```python
from build123d import *

# Parameters (mm, degrees)
BOSS_EXTRUDE1_DEPTH  = 40
SKETCH3_R            = 9
CUT_EXTRUDE1_DEPTH   = 135.350288425
SKETCH4_W            = 25
SKETCH4_H            = 30
CUT_EXTRUDE2_DEPTH   = 30
SKETCH5_R            = 11.1
CUT_EXTRUDE3_DEPTH   = 7
SKETCH6_R            = 11.1
CUT_EXTRUDE4_DEPTH   = 7
CUT_EXTRUDE5_DEPTH   = 41
SKETCH9_W            = 50
SKETCH9_H            = 40
BOSS_EXTRUDE2_DEPTH  = 30
SKETCH11_R           = 1.45
CUT_EXTRUDE8_DEPTH   = 20
SKETCH15_W           = 81.391173049
SKETCH15_H           = 40
SKETCH15_W_2         = 77.391173049
SKETCH15_H_2         = 36
CUT_EXTRUDE9_DEPTH   = 4
SKETCH16_W           = 30
SKETCH16_H           = 40
SKETCH16_W_2         = 26
SKETCH16_H_2         = 36
CUT_EXTRUDE10_DEPTH  = 4
CUT_EXTRUDE11_DEPTH  = 41
SKETCH18_W           = 153.620263659
SKETCH18_H           = 20
BOSS_EXTRUDE3_DEPTH  = 40
CUT_EXTRUDE7_DEPTH   = 41
SKETCH19_W           = 15
SKETCH19_H           = 15
CUT_EXTRUDE12_DEPTH  = 150
SKETCH20_R           = 1.45
CUT_EXTRUDE13_DEPTH  = 20
CUT_EXTRUDE16_DEPTH  = 3
CUT_EXTRUDE18_START  = -7
CUT_EXTRUDE18_DEPTH  = 2.55
SKETCH38_W           = 90
SKETCH38_H           = 20
CUT_EXTRUDE19_DEPTH  = 45.5
CUT_EXTRUDE21_START  = -31.810131
CUT_EXTRUDE21_DEPTH  = 90
BOSS_EXTRUDE11_DEPTH = 40
CHAMFER1_SIZE        = 1.5


with BuildPart() as part:
    # Sketch1 → Boss-Extrude1 (new body)
    with BuildSketch(Plane(origin=(0, 0, 0), x_dir=(1, 0, 0), z_dir=(0, 1, 0))):
        Polygon((-79.503540842, -54.434705768), (-79.503540842, -4.434705768), (-46.700027791, 28.368807283), (-21.951290449, 53.117544624), (-14.880222638, 46.046476813), (-43.164493885, 17.762205565), (-14.880222638, -10.522065682), (13.40404861, 17.762205565), (60.496459158, -29.330204983), (60.496459158, -54.434705768), align=None)
    extrude(amount=BOSS_EXTRUDE1_DEPTH)

    # Sketch3 → Cut-Extrude1 (cut, through all)
    with BuildSketch(Plane(origin=(-37.534417537, 0, -37.534417537), x_dir=(-0.707106781, 0, 0.707106781), z_dir=(-0.707106781, 0, -0.707106781))):
        with Locations((-7.037869671, 20)):
            Circle(SKETCH3_R)
    extrude(amount=-CUT_EXTRUDE1_DEPTH, mode=Mode.SUBTRACT)

    # Sketch4 → Cut-Extrude2 (cut)
    with BuildSketch(Plane(origin=(15.583127088, 0, -15.583127088), x_dir=(-0.707106781, 0, -0.707106781), z_dir=(0.707106781, 0, -0.707106781))):
        with Locations((-19.418317664, 20)):
            Rectangle(SKETCH4_W, SKETCH4_H)
    extrude(amount=-CUT_EXTRUDE2_DEPTH, mode=Mode.SUBTRACT)

    # Sketch5 → Cut-Extrude3 (cut)
    with BuildSketch(Plane(origin=(-37.534417537, 0, -37.534417537), x_dir=(-0.707106781, 0, 0.707106781), z_dir=(-0.707106781, 0, -0.707106781))):
        with Locations((-7.037869671, 20)):
            Circle(SKETCH5_R)
    extrude(amount=-CUT_EXTRUDE3_DEPTH, mode=Mode.SUBTRACT)

    # Sketch6 → Cut-Extrude4 (cut)
    with BuildSketch(Plane(origin=(4.891989334, 0, 4.891989334), x_dir=(0.707106781, 0, -0.707106781), z_dir=(0.707106781, 0, 0.707106781))):
        with Locations(Location((7.037869671, 20, 0), (0, 0, 180))):  # turned: the seam where the file's is
            Circle(SKETCH6_R)
    extrude(amount=-CUT_EXTRUDE4_DEPTH, mode=Mode.SUBTRACT)

    # Sketch7 → Cut-Extrude5 (cut, through all)
    with BuildSketch(Plane(origin=(0, 40, 0), x_dir=(1, 0, 0), z_dir=(0, 1, 0))):
        Polygon((44.116722817, -12.950468642), (44.116722817, -54.434705768), (60.496459158, -54.434705768), (60.496459158, -29.330204983), align=None)
    extrude(amount=-CUT_EXTRUDE5_DEPTH, mode=Mode.SUBTRACT)

    # Sketch9 → Boss-Extrude2 (add)
    with BuildSketch(Plane.ZY.offset(79.503540842)):
        with Locations((29.434705768, 20)):
            Rectangle(SKETCH9_W, SKETCH9_H)
    extrude(amount=BOSS_EXTRUDE2_DEPTH)

    # Sketch11 → Cut-Extrude8 (cut)
    with BuildSketch(Plane(origin=(-37.534417537, 0, -37.534417537), x_dir=(-0.707106781, 0, 0.707106781), z_dir=(-0.707106781, 0, -0.707106781))):
        with Locations((7.962130329, 10)):
            Circle(SKETCH11_R)
        with Locations((7.962130329, 30)):
            Circle(SKETCH11_R)
    extrude(amount=-CUT_EXTRUDE8_DEPTH, mode=Mode.SUBTRACT)

    # Sketch15 → Cut-Extrude9 (cut)
    with BuildSketch(Plane(origin=(-37.534417537, 0, -37.534417537), x_dir=(-0.707106781, 0, 0.707106781), z_dir=(-0.707106781, 0, -0.707106781))):
        with Locations((18.657716854, 20)):
            Rectangle(SKETCH15_W, SKETCH15_H)
        with Locations((18.657716854, 20)):
            Rectangle(SKETCH15_W_2, SKETCH15_H_2, mode=Mode.SUBTRACT)
    extrude(amount=-CUT_EXTRUDE9_DEPTH, mode=Mode.SUBTRACT)

    # Sketch16 → Cut-Extrude10 (cut)
    with BuildSketch(Plane(origin=(0, 0, 4.434705768), x_dir=(-1, 0, 0), z_dir=(0, 0, -1))):
        with Locations((94.503540842, 20)):
            Rectangle(SKETCH16_W, SKETCH16_H)
        with Locations((94.503540842, 20)):
            Rectangle(SKETCH16_W_2, SKETCH16_H_2, mode=Mode.SUBTRACT)
    extrude(amount=-CUT_EXTRUDE10_DEPTH, mode=Mode.SUBTRACT)

    # Sketch17 → Cut-Extrude11 (cut, through all)
    with BuildSketch(Plane.XZ):
        Polygon((-76.675113717, 7.263132892), (-78.089327279, 8.434705768), (-79.503540842, 8.434705768), (-79.503540842, 4.434705768), align=None)
    extrude(amount=-CUT_EXTRUDE11_DEPTH, mode=Mode.SUBTRACT)

    # Sketch18 → Boss-Extrude3 (add)
    with BuildSketch(Plane(origin=(0, 40, 0), x_dir=(1, 0, 0), z_dir=(0, 1, 0))):
        with Locations((-32.693409012, -64.434705768)):
            Rectangle(SKETCH18_W, SKETCH18_H)
    extrude(amount=-BOSS_EXTRUDE3_DEPTH)

    # Sketch10 → Cut-Extrude7 (cut, through all)
    with BuildSketch(Plane(origin=(0, 40, 0), x_dir=(1, 0, 0), z_dir=(0, 1, 0))):
        Polygon((-92.108080814, -70.449971453), (-105.09239053, -54.975873702), (-97.27873721, -48.419440083), (-84.294427494, -63.893537834), align=None)
    extrude(amount=-CUT_EXTRUDE7_DEPTH, mode=Mode.SUBTRACT)

    # Sketch19 → Cut-Extrude12 (cut)
    with BuildSketch(Plane.ZY.offset(109.503540842)):
        with Locations((36.434705768, 20)):
            Rectangle(SKETCH19_W, SKETCH19_H)
    extrude(amount=-CUT_EXTRUDE12_DEPTH, mode=Mode.SUBTRACT)

    # Sketch20 → Cut-Extrude13 (cut)
    with BuildSketch(Plane(origin=(-37.534417537, 0, -37.534417537), x_dir=(-0.707106781, 0, 0.707106781), z_dir=(-0.707106781, 0, -0.707106781))):
        with Locations((45.962130329, 5)):
            Circle(SKETCH20_R)
        with Locations((45.962130329, 35)):
            Circle(SKETCH20_R)
        with Locations((-14.037869671, 35)):
            Circle(SKETCH20_R)
        with Locations((-14.037869671, 5)):
            Circle(SKETCH20_R)
    extrude(amount=-CUT_EXTRUDE13_DEPTH, mode=Mode.SUBTRACT)

    # Sketch36 → Cut-Extrude16 (cut)
    with BuildSketch(Plane(origin=(-30.463349725, 0, -30.463349725), x_dir=(0.707106781, 0, -0.707106781), z_dir=(0.707106781, 0, 0.707106781))):
        Polygon((12.412869671, 37.814582562), (10.787869671, 35), (12.412869671, 32.185417438), (15.662869671, 32.185417438), (17.287869671, 35), (15.662869671, 37.814582562), align=None)
        Polygon((15.662869671, 7.814582562), (12.412869671, 7.814582562), (10.787869671, 5), (12.412869671, 2.185417438), (15.662869671, 2.185417438), (17.287869671, 5), align=None)
        Polygon((-6.337130329, 32.814582562), (-9.587130329, 32.814582562), (-11.212130329, 30), (-9.587130329, 27.185417438), (-6.337130329, 27.185417438), (-4.712130329, 30), align=None)
        Polygon((-6.337130329, 12.814582562), (-9.587130329, 12.814582562), (-11.212130329, 10), (-9.587130329, 7.185417438), (-6.337130329, 7.185417438), (-4.712130329, 10), align=None)
    extrude(amount=-CUT_EXTRUDE16_DEPTH, mode=Mode.SUBTRACT)

    # Sketch37 → Cut-Extrude18 (cut)
    with BuildSketch(Plane(origin=(-37.534417537, 0, -37.534417537), x_dir=(-0.707106781, 0, 0.707106781), z_dir=(-0.707106781, 0, -0.707106781)).offset(CUT_EXTRUDE18_START)):
        Polygon((49.212130329, 5), (49.212130329, 0), (42.712130329, 0), (42.712130329, 5), (44.337130329, 7.814582562), (47.587130329, 7.814582562), align=None)
        Polygon((42.712130329, 35), (44.337130329, 32.185417438), (47.587130329, 32.185417438), (49.212130329, 35), (49.212130329, 40), (42.712130329, 40), align=None)
    extrude(amount=-CUT_EXTRUDE18_DEPTH, mode=Mode.SUBTRACT)

    # Sketch38 → Cut-Extrude19 (cut)
    with BuildSketch(Plane.XY.offset(74.434705768)):
        with Locations((-32.693409012, 20)):
            Rectangle(SKETCH38_W, SKETCH38_H)
    extrude(amount=-CUT_EXTRUDE19_DEPTH, mode=Mode.SUBTRACT)

    # Sketch39 → Cut-Extrude21 (cut)
    with BuildSketch(Plane.ZY.offset(109.503540842).offset(CUT_EXTRUDE21_START)):
        Polygon((28.934705768, 10), (13.968076221, 20), (28.934705768, 30), align=None)
    extrude(amount=-CUT_EXTRUDE21_DEPTH, mode=Mode.SUBTRACT)

    # Sketch42 → Boss-Extrude11 (add)
    with BuildSketch(Plane(origin=(0, 40, 0), x_dir=(1, 0, 0), z_dir=(0, 1, 0))):
        Polygon((-109.503540842, -43.934705768), (-109.503540842, -74.434705768), (-119.503540842, -74.434705768), (-119.503540842, -49.434705768), align=None)
    extrude(amount=-BOSS_EXTRUDE11_DEPTH)

    # Chamfer1
    chamfer1_edges = [part.edges().sort_by_distance(p)[0] for p in [
        (-88.201254154, 0, 67.171754643),
        (-98.600235672, 0, 62.712922577),
        (-101.18556387, 0, 51.697656892),
        (-90.786582352, 0, 56.156488958),
        (-88.201254154, 40, 67.171754643),
        (-90.786582352, 40, 56.156488958),
        (-101.18556387, 40, 51.697656892),
        (-98.600235672, 40, 62.712922577),
    ]]
    chamfer(chamfer1_edges, length=CHAMFER1_SIZE)


solid = part.part
```
Build history of the part. All positions in model axes, mm. A direction names the side the tool comes from. Round coordinates to 2 decimals unless told otherwise and drop trailing zeros. Loops run counter-clockwise (first coordinate to the right, second up) from the corner with the lowest first, then second, coordinate; pieces in that order, holes last.
Item 1: Saw through at A-A (z = 58). List the corners of the cut face in (x, y), then the cut area to 3 significant figures.
Item 2: Saw through at B-B (x = -6). List the corners of the cut face in (y, z), then the cut area to 3 significant figures.
Item 3: Saw through at C-C (x = -50). List the corners of the cut face in (y, z), then the cut area to 3 significant figures.
Item 4: Drill centre lines: line 1 along Y through (x, z) = (-41, 59.5); line 2 along Z through (x, y) = (-47, 37); line 3 along X through (y, z) = (22.5, 11). Where is each one in solid material? Low to high.
Item 5: Which spindle directions (+Z, -Z, +X, -X, +Y, -Y) get a long thin tool onto all of the face, cutting with end or side? Do faces 1 (the face through (-107.504, 20, 6)), 2 (the face through (-77.693, 20, 57)), 3 (the face through (-63.314, 3.094, 1.751)), 4 (the face through (-22, 7.815, -41)). Say none if no direction does.
Item 6: Pin check, flat tips, straight feed: P1, Ø3, axis at y = 4.5, z = 13, coming from the -X side; P2, Ø8, axis at x = -85, y = 22.5, coming from the -Z side; P3, Ø1.2, axis at x = -90, z = 7, coming from the +Y side. Stop position of each tip, or through.
Item 7: Two-plate mould, pull along Y, no slides. Class faces 5 (the face through (-37, 0, 25)), 6 (the face through (-109.504, 20, 26)), 7 (the face through (-33, 10, 52)): released by +Y, released by -Y, zero draft, split by the parting line, or undercut.
Worked answers:
1. outline: (-119.5, 0) - (-104.51, 0) - (-102.55, 1.5) - (-102.55, 38.5) - (-104.51, 40) - (-119.5, 40) - close; (-89.24, 1.5) - (-87.28, 0) - (44.12, 0) - (44.12, 40) - (-87.28, 40) - (-89.24, 38.5) - close; hole (-77.69, 10) - (12.31, 10) - (12.31, 30) - (-77.69, 30) - close
1. area: 4,210 mm2
2. outline: (0, 1.64) - (40, 1.64) - (40, 74.43) - (30, 74.43) - (30, 28.93) - (20, 13.97) - (10, 28.93) - (10, 74.43) - (0, 74.43) - close
2. area: 1,850 mm2
3. outline: (0, -19.41) - (2, -19.41) - (2, -25.07) - (38, -25.07) - (38, -19.41) - (40, -19.41) - (40, 74.43) - (30, 74.43) - (30, 28.93) - (20, 13.97) - (10, 28.93) - (10, 74.43) - (0, 74.43) - close
3. area: 2,900 mm2
4. line 1: y = 0 to 10, 30 to 40
4. line 2: z = -28.07 to 74.43
4. line 3: x = -109.5 to -0.26, 34.14 to 42.17
5. face 1: -Z, -X, +Y, -Y
5. face 2: +Z
5. face 3: -Y
5. face 4: none
6. P1: stops at x = -109.5
6. P2: stops at z = 4.43
6. P3: stops at y = 38
7. face 5: released by -Y
7. face 6: zero draft
7. face 7: undercut
